Source: CAD feature listing. Evaluate the final solid. Frame: model axes, mm. A direction names the side the tool comes from. Coordinates: 2 decimals unless noted, no trailing zeros. Order: outer loops, then holes, each group sorted by start corner. A loop starts at its lowest first (then second) coordinate and runs counter-clockwise, first axis right, second up.
Item 1: Section B-B on x = 42.5. Return the cut outline in (y, z), then the cut area to 3 significant figures.
Item 2: Section A-A on x = 367.5. Return the cut outline in (y, z), then the cut area to 3 significant figures.
Item 3: Ray query, line 1 (Y direction, x = 23.5, z = -1); line 2 (Y direction, x = 456.5, z = 43); line 3 (Z direction, x = 294, y = 17). Return the intervals inside material, ascending.
Item 4: Reachability of faces 1 (the flat face through (508, 1, -1)), 2 (the cylindrical face through (25.756, -4.754, 10.195)) from +Z, -Z, +X, -X, +Y, -Y: full face, straight path, thin tool, end or side. Return the list, or none.
Item 5: Contact query for flat-ended pins moving along their axis: P1, Ø5, axis at x = 198.5, z = 12, coming from the +Y side; P2, Ø12, axis at x = 97.5, y = 12, coming from the +Z side; P3, Ø1, axis at x = 223, y = 29.5, coming from the +Z side. Output: stop coordinate, or through.
from build123d import *

# Parameters (mm, degrees)
SKETCH2_R           = 49.53
BOSS_EXTRUDE1_DEPTH = 152.4
SKETCH3_R           = 12.411567775
BOSS_EXTRUDE2_DEPTH = 50.8


with BuildPart() as part:
    # Sketch1 → Revolve2 (revolve)
    with BuildSketch(Plane(origin=(0, 0, 0), x_dir=(1, 0, 0), z_dir=(0, 1, 0))):
        with BuildLine():
            Line((355.600000053, 50.799999973), (355.600000053, 1.269999973))
            Line((355.600000053, 1.269999973), (50.800000047, 1.269999973))
            Line((50.800000047, 1.269999973), (50.800000047, 13.68156774))
            add(Edge.make_bspline(
                [(50.800000047, 13.68156774), (51.224607869, 13.786541703), (52.079748124, 13.99736018), (53.901316113, 14.445024847), (55.90428978, 14.933081433), (57.918204029, 15.420277853), (59.969167456, 15.913068852), (62.005618607, 16.398707152), (64.04585603, 16.881716673), (66.619566178, 17.486536085), (69.727395203, 18.209576077), (73.370678613, 19.04644661), (77.55044141, 19.991710093), (82.779136229, 21.155661521), (97.433989811, 24.348822924), (119.485629173, 28.81699746), (168.00075752, 37.516041455), (219.035004801, 44.081341124), (262.822405655, 47.820230422), (299.206459448, 49.570692635), (308.841173655, 49.947366018), (315.265578413, 50.162354186), (319.548981494, 50.29122703), (323.832782669, 50.405645805), (328.116966628, 50.505609209), (332.401425999, 50.591116104), (336.139078075, 50.653092889), (339.329601827, 50.697064227), (341.973247658, 50.727612371), (344.069774299, 50.748376802), (346.163273231, 50.76568058), (348.272494467, 50.77952366), (350.344714481, 50.789906003), (352.405704949, 50.79682758), (354.282013928, 50.799423175), (355.162608625, 50.799999974), (355.600000053, 50.799999973)],
                knots=[0.08282658, 0.08282658, 0.08282658, 0.08282658, 0.08282658, 0.088510594, 0.094194608, 0.099878623, 0.105562637, 0.111246651, 0.116930666, 0.12261468, 0.128298694, 0.139917182, 0.15153567, 0.163154157, 0.174772645, 0.198009616, 0.314194483, 0.407142375, 0.709223026, 0.755696971, 0.790552431, 0.802170918, 0.813789405, 0.825407891, 0.837026378, 0.848644864, 0.860263351, 0.871881838, 0.877565852, 0.883249866, 0.88893388, 0.894617894, 0.900301908, 0.905985922, 0.911669936, 0.91735395, 0.91735395, 0.91735395, 0.91735395, 0.91735395], degree=4))
        make_face()
    revolve(axis=Axis((355.600000053, 0, -1.269999973), (-1, 0, 0)))

    # Sketch2 → Boss-Extrude1 (add)
    with BuildSketch(Plane(origin=(355.600000053, 0, 0), x_dir=(0, 0, -1), z_dir=(1, 0, 0))):
        with Locations((1.269999973, 0)):
            Circle(SKETCH2_R)
    extrude(amount=BOSS_EXTRUDE1_DEPTH)

    # Sketch3 → Boss-Extrude2 (add)
    with BuildSketch(Plane.ZY.offset(-50.800000063)):
        with Locations((-1.269999973, 0)):
            Circle(SKETCH3_R)
    extrude(amount=BOSS_EXTRUDE2_DEPTH)


solid = part.part
Answer list:
1. outline: circle Ø24.82 at (0, -1.27)
1. area: 484 mm2
2. outline: circle Ø99.06 at (0, -1.27)
2. area: 7,710 mm2
3. line 1: y = -12.41 to 12.41
3. line 2: y = -22.21 to 22.21
3. line 3: z = -46.2 to 43.66
4. face 1: +Z, -Z, +X, +Y, -Y
4. face 2: -X
5. P1: stops at y = 38.36
5. P2: stops at z = 21.38
5. P3: stops at z = 29.93
